Can you work these out from the drawing? Everything is in mm from the part's minimum corner. A direction names the side the tool comes from. Coordinates: 2 decimals unless noted, no trailing zeros. Order: outer loops, then holes, each group sorted by start corner. A loop starts at its lowest first (then second) coordinate and runs counter-clockwise, first axis right, second up. Notation, with made-up numbers: (21.5, 58.5) -> (41.5, 58.5) arc R22 cw to (41.5, 92.5) -> close; hole circle Ø1 at (-34.75, 65). An arc over 180 degrees is marked (long way). Return JSON: item names as keys, results as strings. Group by question number.
1) If we section it at B-B, the plane z = 5: Please give me the cut outline in (x, y), then the cut area to 3 significant figures.
2) If we section it at D-D, the plane y = 5.5: Please give me the cut outline in (x, z), then the cut area to 3 significant figures.
3) For pin 1 (1.5 mm diameter, centred on x = 111, z = 5, fed in from +Y); pin 2 (3 mm diameter, centred on x = 129, z = 5, fed in from +Y); pin 3 (2 mm diameter, centred on x = 59, y = 4.5, fed in from -Z), each with a flat end and sliding along its axis, tell me the tip position at first contact or that it passes through.
4) For the marked faces 1 and 2, which set-ups out of +Z, -Z, +X, -X, +Y, -Y let a thin tool reach every point of the face, with its end or its side?
5) If we section it at A-A, the plane x = 129: Please give me the cut outline in (y, z).
6) If we section it at C-C, the plane x = 58: Please give me the cut outline in (y, z).
7) If I drill on probe 1 along X at (y, z) = (1.1, 5); probe 2 along Z at (x, y) = (24, 2); probe 3 along Y at (x, z) = (118, 10.75), over which ranges is the centre line in solid material (lowest first)? Write a range as from..to.
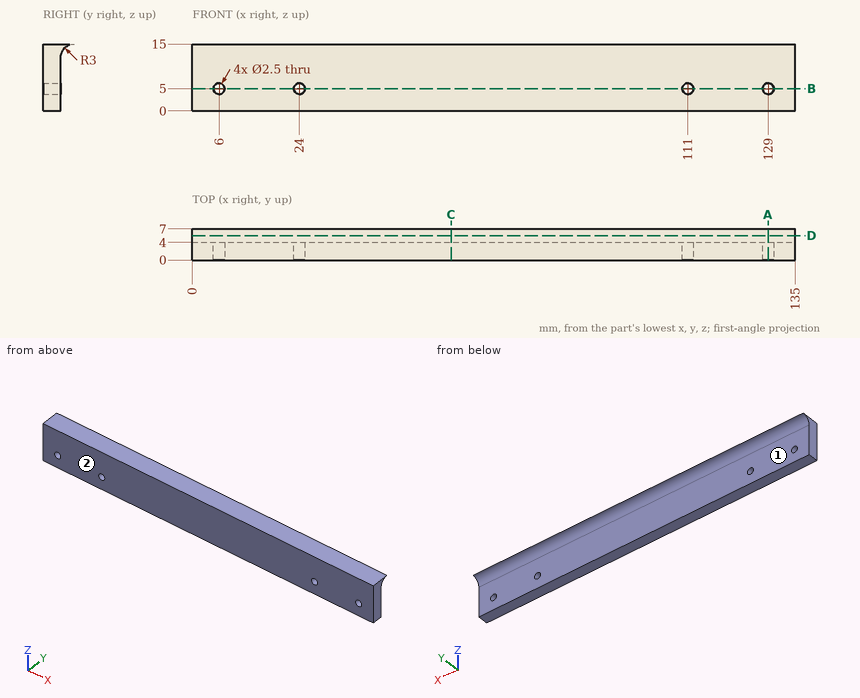
Result sheet:
{
 "1": {"outline": "(0, 0) -> (4.75, 0) -> (4.75, 4) -> (0, 4) -> close; (7.25, 0) -> (22.75, 0) -> (22.75, 4) -> (7.25, 4) -> close; (25.25, 0) -> (109.75, 0) -> (109.75, 4) -> (25.25, 4) -> close; (112.25, 0) -> (127.75, 0) -> (127.75, 4) -> (112.25, 4) -> close; (130.25, 0) -> (135, 0) -> (135, 4) -> (130.25, 4) -> close", "area": "500 mm2"},
 "2": {"outline": "(0, 14.6) -> (135, 14.6) -> (135, 15) -> (0, 15) -> close", "area": "54.3 mm2"},
 "3": {"pin 1": "passes through", "pin 2": "stops at y = 4", "pin 3": "stops at z = 0"},
 "4": {"face 1": "-Z, +X, -X, +Y", "face 2": "+Z, -Z, +X, -X, -Y"},
 "5": {"outline": "(0, 0) -> (4, 0) -> (4, 3.75) -> (0, 3.75) -> close; (0, 6.25) -> (4, 6.25) -> (4, 12) arc R3 cw to (7, 15) -> (0, 15) -> close"},
 "6": {"outline": "(0, 0) -> (4, 0) -> (4, 12) arc R3 cw to (7, 15) -> (0, 15) -> close"},
 "7": {"probe 1": "x = 0..4.75, 7.25..22.75, 25.25..109.75, 112.25..127.75, 130.25..135", "probe 2": "z = 0..3.75, 6.25..15", "probe 3": "y = 0..4"}
}
